Study the drawing (mm; zero at the part's minimum x, y, z) and answer. A direction names the side the tool comes from. Coordinates: 2 decimals unless noted, no trailing zeros. Loops run counter-clockwise (first coordinate to the right, second up) from the corner with the lowest first, then second, coordinate; pieces in that order, holes last.
Q1. Section A-A (x = 30.94) is taken. Give the vertices of the cut face in (y, z).
Q2. Which of the six approach directions +Z, -Z, +X, -X, +Y, -Y give full straight-line access (tool end or side, diameter ignored) to the marked faces 4, 5, 6 and 7?
Q3. The mould has two halves that part along Y. Classify the marked faces 1, 2 and 3: pulls with the +Y half, pulls with the -Y half, needs draft (parallel to the pull), parting line crosses it, or undercut.
Q4. Flat-ended cylindrical pins translate along their axes: P1, Ø2, axis at y = 20.5, z = 3.5, coming from the +X side; P2, Ø5, axis at x = 28, y = 24, coming from the +Z side; P3, Ø1.9, axis at x = 26, z = 9, coming from the +Y side; P4, Ø1.3, axis at y = 21, z = 6.5, coming from the -X side. Find the tip coordinate at first contact, or state that the pin passes through.
Q5. Section C-C (x = 17) is taken. Give the vertices of the cut face in (y, z), then the cut area to 3 significant figures.
Q6. Straight lines are drawn through the part: line 1 (Z direction, x = 30.94, y = 17.5); line 2 (Y direction, x = 22, z = 2); line 3 (X direction, y = 9, z = 9). For each, find the intervals that lie inside material, in ascending order.
Q7. Section B-B (y = 14.5) is taken. Give the vertices of the cut face in (x, z).
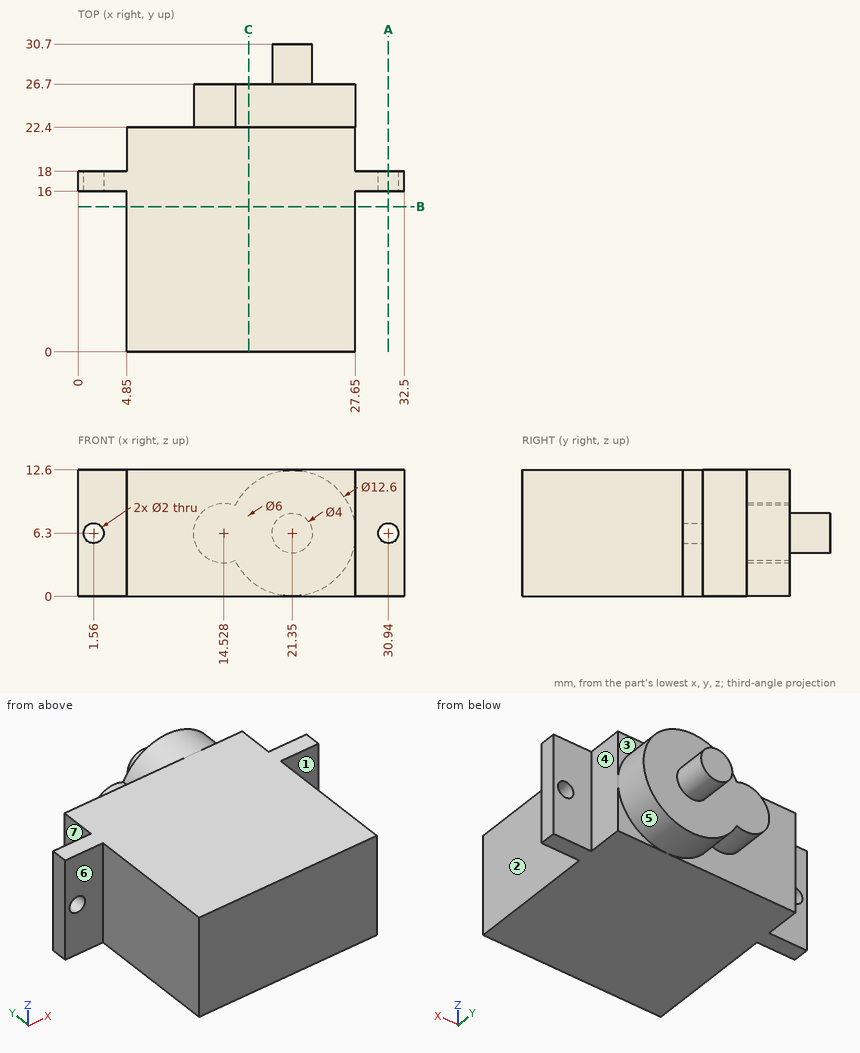
Numbers:
1. outline: (16, 0) - (18, 0) - (18, 5.3) - (16, 5.3) - close; (16, 7.3) - (18, 7.3) - (18, 12.6) - (16, 12.6) - close
2. face 4: +Z, -Z, +X, +Y
2. face 5: +Y
2. face 6: +Z, -Z, -X, -Y
2. face 7: +Z, -Z, -X, +Y
3. face 1: pulls with the -Y half
3. face 2: needs draft
3. face 3: pulls with the +Y half
4. P1: stops at x = 27.65
4. P2: stops at z = 12.6
4. P3: stops at y = 26.7
4. P4: stops at x = 4.85
5. outline: (0, 0) - (22.4, 0) - (22.4, 1.74) - (26.7, 1.74) - (26.7, 10.86) - (22.4, 10.86) - (22.4, 12.6) - (0, 12.6) - close
5. area: 321 mm2
6. line 1: z = 0 to 5.3, 7.3 to 12.6
6. line 2: y = 0 to 26.7
6. line 3: x = 4.85 to 27.65
7. outline: (4.85, 0) - (27.65, 0) - (27.65, 12.6) - (4.85, 12.6) - close
